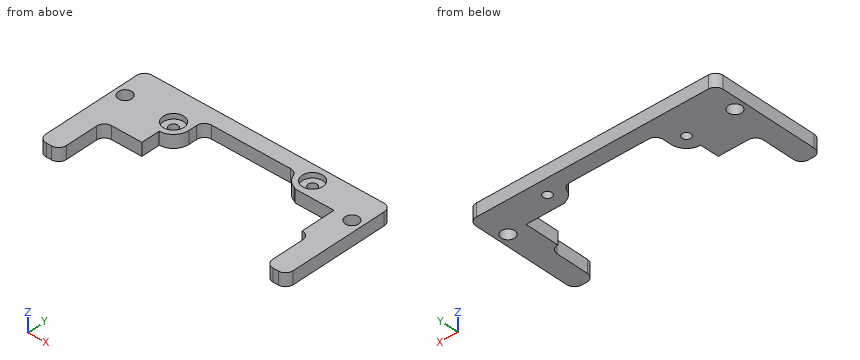
```python
from build123d import *

# Parameters (mm, degrees)
ESQUISSE1_R             = 2.6
ESQUISSE1_R_2           = 1.7
BOSS_EXTRU_1_DEPTH      = 5
ESQUISSE2_R             = 4
ENL_V_MAT_EXTRU_1_DEPTH = 2
ENL_V_MAT_EXTRU_2_DEPTH = 5


with BuildPart() as part:
    # Esquisse1 → Boss.-Extru.1 (new body)
    with BuildSketch(Plane.XY):
        with BuildLine():
            Line((7, -13.31223453), (81, -13.31223453))
            ThreePointArc((81, -13.31223453), (83.121320344, -14.190914186), (84, -16.31223453))
            Line((84, -16.31223453), (84, -29))
            ThreePointArc((84, -29), (84.878679656, -31.121320344), (87, -32))
            Line((87, -32), (89, -32))
            ThreePointArc((89, -32), (91.121320344, -31.121320344), (92, -29))
            Line((92, -29), (92, 9.22))
            ThreePointArc((92, 9.22), (91.121320344, 11.341320344), (89, 12.22))
            Line((89, 12.22), (-1, 12.22))
            ThreePointArc((-1, 12.22), (-3.121320344, 11.341320344), (-4, 9.22))
            Line((-4, 9.22), (-4, -29))
            ThreePointArc((-4, -29), (-3.121320344, -31.121320344), (-1, -32))
            Line((-1, -32), (1, -32))
            ThreePointArc((1, -32), (3.121320344, -31.121320344), (4, -29))
            Line((4, -29), (4, -16.31223453))
            ThreePointArc((4, -16.31223453), (4.878679656, -14.190914186), (7, -13.31223453))
        make_face()
        Circle(ESQUISSE1_R, mode=Mode.SUBTRACT)
        with Locations((88, 0)):
            Circle(ESQUISSE1_R, mode=Mode.SUBTRACT)
        with Locations((18.779545265, 0)):
            Circle(ESQUISSE1_R_2, mode=Mode.SUBTRACT)
        with Locations((66.979545265, 6.22)):
            Circle(ESQUISSE1_R_2, mode=Mode.SUBTRACT)
    extrude(amount=BOSS_EXTRU_1_DEPTH)

    # Esquisse2 → Enlèv. mat.-Extru.1 (cut)
    with BuildSketch(Plane.XY.offset(5)):
        with Locations((18.779545265, 0)):
            Circle(ESQUISSE2_R)
        with Locations((66.979545265, 6.22)):
            Circle(ESQUISSE2_R)
    extrude(amount=-ENL_V_MAT_EXTRU_1_DEPTH, mode=Mode.SUBTRACT)

    # Esquisse3 → Enlèv. mat.-Extru.2 (cut)
    with BuildSketch(Plane.XY.offset(5)):
        with BuildLine():
            Line((18.779545265, -6), (18.779545265, -10.31223453))
            Line((18.779545265, -10.31223453), (18.779545265, -13.31223453))
            Line((18.779545265, -13.31223453), (21.779545265, -13.31223453))
            Line((21.779545265, -13.31223453), (63.979545265, -13.31223453))
            Line((63.979545265, -13.31223453), (81, -13.31223453))
            Line((81, -13.31223453), (81, 0))
            Line((81, 0), (65.946395614, 0))
            ThreePointArc((65.946395614, 0), (65.489457028, 0.327047013), (64.979545265, 0.563145751))
            ThreePointArc((64.979545265, 0.563145751), (62.736904578, 1.977359313), (61.322691016, 4.22))
            ThreePointArc((61.322691016, 4.22), (60.226314699, 5.669489743), (58.494263891, 6.22))
            Line((58.494263891, 6.22), (27.779545265, 6.22))
            ThreePointArc((27.779545265, 6.22), (25.658224922, 5.341320344), (24.779545265, 3.22))
            Line((24.779545265, 3.22), (24.779545265, 0))
            ThreePointArc((24.779545265, 0), (23.022185952, -4.242640687), (18.779545265, -6))
        make_face()
    extrude(amount=-ENL_V_MAT_EXTRU_2_DEPTH, mode=Mode.SUBTRACT)


solid = part.part
```
Source: CAD feature listing. Evaluate the final solid. Frame: model axes, mm. Coordinates: 2 decimals unless noted, no trailing zeros. Write each loop counter-clockwise with the first axis right and the second up, starting at its lowest first coordinate (ties: lowest second). Pieces come first, ordered by that corner, then holes. Notation, with made-up numbers: M -23.75,78.25 L 18.25,78.25 A24 cw 18.25,101.25 Z; hole C -36,46 d7. An arc over 180 degrees is marked long. Answer as a JSON object with one key per item and string values.
1. Ray query, L1, parallel to X at y = -10, z = 4.65; L2, parallel to X at y = -1, z = 0.5; L3, parallel to Y at x = 88, z = 1.4. Return the intervals inside material, ascending.
Evaluation:
{"L1": "-4 to 18.78, 81 to 92", "L2": "-4 to -2.4, 2.4 to 17.4, 20.15 to 24.7, 81 to 85.6, 90.4 to 92", "L3": "-32 to -2.6, 2.6 to 12.22"}
2. Cut plane A-A on y = -23.5. Output: boundary loops of the cut face in (x, z), plus the area to 3 significant figures.
Evaluation:
{"outline": "M -4,0 L 4,0 L 4,5 L -4,5 Z; M 84,0 L 92,0 L 92,5 L 84,5 Z", "area": "80.0 mm^2"}
3. Cut plane D-D on x = 49.5. Output: boundary loops of the cut face in (y, z).
Evaluation:
{"outline": "M 6.22,0 L 12.22,0 L 12.22,5 L 6.22,5 Z"}
4. Cut plane B-B on z = 1.95. State how many separate pieces and enclosed holes the cut face has, plus the area to 3 significant figures.
Evaluation:
{"separate pieces": "1", "enclosed holes": "4", "area": "1,650 mm^2"}
5. Contact query for flat-ended pins moving along their axis: P1, Ø3, axis at x = 13.5, z = 3, coming from the -Y side; P2, Ø5, axis at x = 66.98, y = 6.22, coming from the +Z side; P3, Ø3, axis at x = 18.78, y = 0, coming from the -Z side; P4, Ø1.5, axis at x = 74, z = 3, coming from the -Y side. Output: stop coordinate, or through.
Evaluation:
{"P1": "y = -13.31", "P2": "z = 3", "P3": "through", "P4": "y = 0"}
6. Cut plane C-C on x = 0. Output: boundary loops of the cut face in (y, z).
Evaluation:
{"outline": "M -32,0 L -2.6,0 L -2.6,5 L -32,5 Z; M 2.6,0 L 12.22,0 L 12.22,5 L 2.6,5 Z"}
